```python
from build123d import *

# Parameters (mm, degrees)
AUFSATZ_LINEAR_AUSTRAGEN1_DEPTH      = 19
SKIZZE3_W                            = 156.5
SKIZZE3_H                            = 16.8
AUFSATZ_LINEAR_AUSTRAGEN2_DEPTH      = 19
SCHNITT_LINEAR_AUSTRAGEN1_DEPTH      = 19
SCHNITT_LINEAR_AUSTRAGEN1_DEPTH_BACK = 19
BOHRUNG1_D                           = 10
BOHRUNG2_D                           = 8.566
BOHRUNG2_DEPTH                       = 8.5
BOHRUNG2_CSINK_D                     = 9.728
BOHRUNG2_CSINK_ANGLE                 = 90
BOHRUNG3_D                           = 8.566
BOHRUNG3_DEPTH                       = 8.5
BOHRUNG3_CSINK_D                     = 9.728
BOHRUNG3_CSINK_ANGLE                 = 90


with BuildPart() as part:
    # Skizze1 → Rotation1 (revolve)
    with BuildSketch(Plane.XY, mode=Mode.PRIVATE) as rotation1_sk:
        with BuildLine():
            Line((0, 0), (0, 13.3))
            Line((0, 13.3), (0.6, 13.9))
            Line((0.6, 13.9), (3, 13.9))
            Line((3, 13.9), (4.1, 15))
            Line((4.1, 15), (20.95, 15))
            Line((20.95, 15), (21.865685425, 14.084314575))
            ThreePointArc((21.865685425, 14.084314575), (22.125224104, 13.910896374), (22.43137085, 13.85))
            Line((22.43137085, 13.85), (23.2, 13.85))
            ThreePointArc((23.2, 13.85), (23.765685425, 14.084314575), (24, 14.65))
            Line((24, 14.65), (24, 15))
            Line((24, 15), (26, 15))
            Line((26, 15), (26, 0))
            Line((26, 0), (0, 0))
        make_face()
    revolve(rotation1_sk.sketch.rotate(Axis((26, 0, 0), (-1, 0, 0)), 270), axis=Axis((26, 0, 0), (-1, 0, 0)))

    # Skizze2 → Aufsatz-Linear austragen1 (add)
    with BuildSketch(Plane(origin=(26, 0, 0), x_dir=(0, 0, -1), z_dir=(1, 0, 0))):
        with BuildLine():
            Line((8.6, 17.125419703), (8.6, 18.8))
            ThreePointArc((8.6, 18.8), (8.541421356, 18.941421356), (8.4, 19))
            Line((8.4, 19), (-8.4, 19))
            ThreePointArc((-8.4, 19), (-8.541421356, 18.941421356), (-8.6, 18.8))
            Line((-8.6, 18.8), (-8.6, 17.125419703))
            ThreePointArc((-8.6, 17.125419703), (-8.643579842, 16.969699754), (-8.761658017, 16.859221476))
            ThreePointArc((-8.761658017, 16.859221476), (-8e-09, -19), (8.761658031, 16.859221469))
            ThreePointArc((8.761658031, 16.859221469), (8.643579846, 16.969699747), (8.6, 17.125419703))
        make_face()
    extrude(amount=AUFSATZ_LINEAR_AUSTRAGEN1_DEPTH)

    # Skizze3 → Rotation2 (revolve)
    with BuildSketch(Plane.XY, mode=Mode.PRIVATE) as rotation2_sk:
        with Locations((123.25, 8.4)):
            Rectangle(SKIZZE3_W, SKIZZE3_H)
    revolve(rotation2_sk.sketch.rotate(Axis((201.5, 0, 0), (-1, 0, 0)), 270), axis=Axis((201.5, 0, 0), (-1, 0, 0)))

    # Skizze4 → Aufsatz-Linear austragen2 (add)
    with BuildSketch(Plane(origin=(201.5, 0, 0), x_dir=(0, 0, -1), z_dir=(1, 0, 0))):
        with BuildLine():
            Line((8.6, 17.125419703), (8.6, 18.8))
            ThreePointArc((8.6, 18.8), (8.541421356, 18.941421356), (8.4, 19))
            Line((8.4, 19), (-8.4, 19))
            ThreePointArc((-8.4, 19), (-8.541421356, 18.941421356), (-8.6, 18.8))
            Line((-8.6, 18.8), (-8.6, 17.125419703))
            ThreePointArc((-8.6, 17.125419703), (-8.643579842, 16.969699754), (-8.761658017, 16.859221476))
            ThreePointArc((-8.761658017, 16.859221476), (-8e-09, -19), (8.761658031, 16.859221469))
            ThreePointArc((8.761658031, 16.859221469), (8.643579846, 16.969699747), (8.6, 17.125419703))
        make_face()
    extrude(amount=AUFSATZ_LINEAR_AUSTRAGEN2_DEPTH)

    # Skizze5 → Rotation3 (revolve)
    with BuildSketch(Plane.XY, mode=Mode.PRIVATE) as rotation3_sk:
        with BuildLine():
            Line((220.5, 0), (220.5, 15))
            Line((220.5, 15), (222.5, 15))
            Line((222.5, 15), (222.5, 14.65))
            ThreePointArc((222.5, 14.65), (222.734314575, 14.084314575), (223.3, 13.85))
            Line((223.3, 13.85), (224.06862915, 13.85))
            ThreePointArc((224.06862915, 13.85), (224.374775896, 13.910896374), (224.634314575, 14.084314575))
            Line((224.634314575, 14.084314575), (225.55, 15))
            Line((225.55, 15), (242.4, 15))
            Line((242.4, 15), (243.5, 13.9))
            Line((243.5, 13.9), (245.9, 13.9))
            Line((245.9, 13.9), (246.5, 13.3))
            Line((246.5, 13.3), (246.5, 0))
            Line((246.5, 0), (220.5, 0))
        make_face()
    revolve(rotation3_sk.sketch.rotate(Axis((246.5, 0, 0), (-1, 0, 0)), 270), axis=Axis((246.5, 0, 0), (-1, 0, 0)))

    # Skizze6 → Schnitt-Linear austragen1 (cut, two sides: drawn at the far end of the back side and taken through both)
    with BuildSketch(Plane(origin=(0, 0, 0), x_dir=(1, 0, 0), z_dir=(0, 1, 0)).offset(-SCHNITT_LINEAR_AUSTRAGEN1_DEPTH_BACK)):
        Polygon((221.5, 24), (221.5, 8), (246.5, 8), (246.5, -8), (221.5, -8), (221.5, -24), (262.5, -24), (262.5, 24), align=None)
    extrude(amount=SCHNITT_LINEAR_AUSTRAGEN1_DEPTH + SCHNITT_LINEAR_AUSTRAGEN1_DEPTH_BACK, mode=Mode.SUBTRACT)

    # Bohrung1 (through all)
    with Locations(Plane(origin=(0, 0, -8), x_dir=(-1, 0, 0), z_dir=(0, 0, -1))):
        with Locations((-234.5, 0)):
            Hole(BOHRUNG1_D / 2)

    # Bohrung2
    with Locations(Plane(origin=(0, 19, 0), x_dir=(1, 0, 0), z_dir=(0, 1, 0))):
        with Locations((35, 0)):
            CounterSinkHole(BOHRUNG2_D / 2, BOHRUNG2_CSINK_D / 2, depth=BOHRUNG2_DEPTH, counter_sink_angle=BOHRUNG2_CSINK_ANGLE)

    # Bohrung3
    with Locations(Plane(origin=(0, 19, 0), x_dir=(1, 0, 0), z_dir=(0, 1, 0))):
        with Locations((211.5, 0)):
            CounterSinkHole(BOHRUNG3_D / 2, BOHRUNG3_CSINK_D / 2, depth=BOHRUNG3_DEPTH, counter_sink_angle=BOHRUNG3_CSINK_ANGLE)

    # Skizze13 → Schnitt-Rotation1 (revolve, cut)
    with BuildSketch(Plane.XY, mode=Mode.PRIVATE) as schnitt_rotation1_sk:
        Polygon((-8, 0), (-8, 6), (57, 6), (57, 16), (190, 16), (190, 0), align=None)
    revolve(schnitt_rotation1_sk.sketch.rotate(Axis((190, 0, 0), (-1, 0, 0)), 270), axis=Axis((190, 0, 0), (-1, 0, 0)), mode=Mode.SUBTRACT)


solid = part.part
```
The model under review builds one solid part; all positions refer to its coordinate system, in mm. A direction names the side the tool comes from. Coordinates: 2 decimals unless noted, no trailing zeros. Write each loop counter-clockwise with the first axis right and the second up, starting at its lowest first coordinate (ties: lowest second). Pieces come first, ordered by that corner, then holes.
1) To check wall thickness, follow probe 1 along Y at (x, z) = (148, 7.5); probe 2 along Y at (x, z) = (40, 0.5); probe 3 along X at (y, z) = (-4, 11). State the ranges of each line that lie inside material, in increasing order.
2) Machinability: for faces 4 (the face through (12.643, 0.66, -14.985)), 5 (the face through (234, 15, 0)), 6 (the face through (228, 0, -8)), 7 (the face through (35, 10.5, 0)), 8 (the face through (234, -15, 0)), which of the approach directions +Z, -Z, +X, -X, +Y, -Y give a long, thin tool a straight path to every point of the face, cutting with its end or side? Answer none if there is none.
3) We need section A-A on x = 234.5. State the section outline as (y, z) points.
4) We need section B-B on x = 35. State the section outline as (y, z) points.
5) We need section C-C on x = 197. State the section outline as (y, z) points.
6) The part is to be moulded in two halves that separate along X. For faces 1 (the face through (40, 19, -2)), 2 (the face through (26, 13, -8)), 3 (the face through (124.43, -15.62, -3.47)), say which applies: pulls with the +X half, pulls with the -X half, needs draft (parallel to the pull), parting line crosses it, or undercut.
7) We need section D-D on x = 68. State the section outline as (y, z) points, then the cut area to 3 significant figures.
8) Clearance check with flat-ended pins moving along their axes: pin 1 Ø3.5 at (y, z) = (-2, 12.5) entering from +X; pin 2 Ø1.5 at (x, y) = (184.5, 9) entering from +Z; pin 3 Ø9 at (x, y) = (234.5, 0) entering from +Z; pin 4 Ø1.8 at (x, y) = (211, 18) entering from -Z. State where each tip first meets the part, or that it passes through.
Answer list:
1. probe 1: y = -15.03 to -14.13, 14.13 to 15.03
1. probe 2: y = -18.99 to -5.98, 5.98 to 19
1. probe 3: x = 0 to 57, 190 to 221.5
2. face 4: -X
2. face 5: +X, +Y
2. face 6: -Z, +X, +Y, -Y
2. face 7: +Y
2. face 8: +X, -Y
3. outline: (-12.69, -8) - (-5, -8) - (-5, 8) - (-12.69, 8) arc R15 ccw to start; (5, -8) - (12.69, -8) arc R15 ccw to (12.69, 8) - (5, 8) - close
4. outline: (10.5, -4.28) - (10.5, 4.28) - (18.42, 4.28) - (19, 4.86) - (19, 8.4) arc R0.2 ccw to (18.8, 8.6) - (17.13, 8.6) arc R0.3 cw to (16.86, 8.76) arc R19 ccw (long way) to (16.86, -8.76) arc R0.3 cw to (17.13, -8.6) - (18.8, -8.6) arc R0.2 ccw to (19, -8.4) - (19, -4.86) - (18.42, -4.28) - close; hole circle Ø12 at (0, 0)
5. outline: circle Ø33.6 at (0, 0)
6. face 1: needs draft
6. face 2: pulls with the -X half
6. face 3: undercut
7. outline: circle Ø33.6 at (0, 0); hole circle Ø32 at (0, 0)
7. area: 82.4 mm2
8. pin 1: stops at x = 221.5
8. pin 2: stops at z = 14.63
8. pin 3: passes through
8. pin 4: stops at z = -8.6
